```python
from build123d import *

# Parameters (mm, degrees)
SKETCH1_R           = 3.5
SKETCH1_R_2         = 1.5
BOSS_EXTRUDE1_DEPTH = 2
FILLET2_R           = 5
SKETCH2_R           = 5.5
SKETCH2_R_2         = 1.235500329
BOSS_EXTRUDE2_DEPTH = 5
FILLET3_R           = 2
CUT_EXTRUDE1_START  = -5
SKETCH3_R           = 3
CUT_EXTRUDE1_DEPTH  = 4


with BuildPart() as part:
    # Sketch1 → Boss-Extrude1 (new body)
    with BuildSketch(Plane(origin=(0, 0, 0), x_dir=(1, 0, 0), z_dir=(0, 1, 0))):
        Polygon((0, 6.5), (-22.384997637, 4.939274727), (-22.384997637, -5.060725273), (0, -6.5), (21.514033914, -5), (21.514033914, 5), align=None)
        with Locations(Location((0, 0, 0), (0, 0, 270))):
            Circle(SKETCH1_R, mode=Mode.SUBTRACT)
        with Locations(Location((-18, 0, 0), (0, 0, 270))):
            Circle(SKETCH1_R_2, mode=Mode.SUBTRACT)
        with Locations(Location((18, 0, 0), (0, 0, 270))):
            Circle(SKETCH1_R_2, mode=Mode.SUBTRACT)
    extrude(amount=BOSS_EXTRUDE1_DEPTH)

    # Fillet2
    fillet2_edges = [part.edges().sort_by_distance(p)[0] for p in [
        (-22.384997637, 1, 5.060725273),
        (-22.384997637, 1, -4.939274727),
        (21.514033914, 1, -5),
        (21.514033914, 1, 5),
    ]]
    fillet(fillet2_edges, radius=FILLET2_R)

    # Sketch2 → Boss-Extrude2 (add)
    with BuildSketch(Plane(origin=(0, 0, 0), x_dir=(1, 0, 0), z_dir=(0, 1, 0))):
        with Locations(Location((0, 0, 0), (0, 0, 270))):
            Circle(SKETCH2_R)
        with Locations(Location((0, 0, 0), (0, 0, 270))):
            Circle(SKETCH2_R_2, mode=Mode.SUBTRACT)
    extrude(amount=-BOSS_EXTRUDE2_DEPTH)

    # Fillet3
    # the kernel refuses this fillet: 2 mm, written as the material it adds along each edge
    with BuildSketch(Plane(origin=(0, 0, 0), x_dir=(0, 0, 1), z_dir=(-1, 0, 0))) as fillet3_piece_1_section:
        with BuildLine():
            CenterArc((5.5 + FILLET3_R, -FILLET3_R), FILLET3_R, 90, 90)
            Line((5.5, -FILLET3_R), (5.5, 0))
            Line((5.5, 0), (5.5 + FILLET3_R, 0))
        make_face()
    fillet3_piece_1 = revolve(axis=Axis((0, 0, 0), (0, 1, 0)), mode=Mode.PRIVATE)
    fillet3_piece_1 = split(fillet3_piece_1, bisect_by=Plane(origin=(-0.030373147, -0.562249721, -6.497882326), z_dir=(0.06955308260096395, 0, 0.9975782519184666)), keep=Keep.TOP, mode=Mode.PRIVATE)
    fillet3_piece_1 = split(fillet3_piece_1, bisect_by=Plane(origin=(0.030373147, -0.562249721, -6.497882326), z_dir=(-0.06955308260096384, 0, 0.9975782519184666)), keep=Keep.TOP, mode=Mode.PRIVATE)
    fillet3_piece_1 = split(fillet3_piece_1, bisect_by=Plane(origin=(-0.804382076, -0.562249721, 6.44828113), z_dir=(0.06416390756024656, 0, -0.9979393733922919)), keep=Keep.TOP, mode=Mode.PRIVATE)
    fillet3_piece_1 = split(fillet3_piece_1, bisect_by=Plane(origin=(0.871627207, -0.562249721, 6.439228468), z_dir=(-0.06955308260096384, 0, -0.9975782519184666)), keep=Keep.TOP, mode=Mode.PRIVATE)
    add(fillet3_piece_1)

    # Sketch3 → Cut-Extrude1 (cut)
    with BuildSketch(Plane(origin=(0, 0, 0), x_dir=(1, 0, 0), z_dir=(0, 1, 0)).offset(CUT_EXTRUDE1_START)):
        with Locations(Location((0, 0, 0), (0, 0, 270))):
            Circle(SKETCH3_R)
    extrude(amount=CUT_EXTRUDE1_DEPTH, mode=Mode.SUBTRACT)


solid = part.part
```
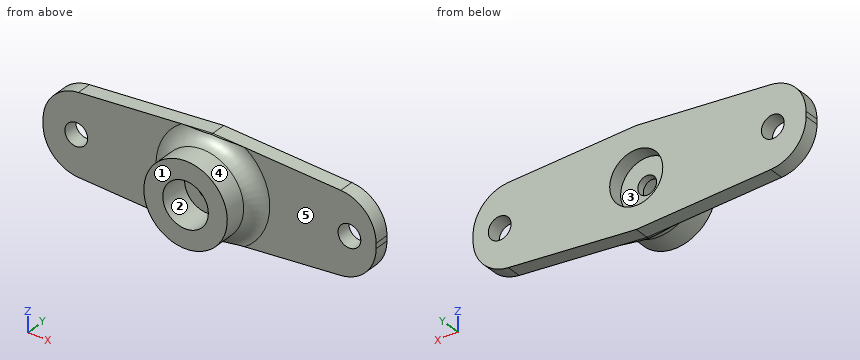
Could you check a few things on this model? Use its own coordinates, in mm. Face numbers are marked on the shaded views. A direction names the side the tool comes from. Give positions to 0.01 mm unless a question says otherwise; leave off trailing zeros. Write each loop counter-clockwise with the first axis right and the second up, starting at its lowest first coordinate (ties: lowest second). Pieces come first, ordered by that corner, then holes. Notation, with made-up numbers: (38.25, 17.5) -> (94.25, 17.5) arc R14 cw to (94.25, 42.5) -> close; hole circle Ø4 at (24.25, 31). An arc over 180 degrees is marked (long way). Write each question's results on one line, items separated by ' | '.
1. If we mould it in two halves opening along X, with no side actions, what happens to the marked faces 3, 4 and 5? For each: released by +X, released by -X, zero draft, split by the parting line, or undercut.
Check sheet entries:
face 3: undercut | face 4: split by the parting line | face 5: zero draft
2. Will these pins go through, and if not, where does the flat tip stop? pin 1 Ø6.5 at (x, z) = (0, 0) entering from -Y; pin 2 Ø2 at (x, y) = (16.5, -1.5) entering from -Z; pin 3 Ø5.5 at (x, z) = (0, 0) entering from -Y; pin 4 Ø4 at (x, z) = (0, 0) entering from +Y.
Check sheet entries:
pin 1: stops at y = -5 | pin 2: passes through | pin 3: stops at y = -1 | pin 4: stops at y = 0
3. I want a section at B-B, the plane x = -19. Write out the boundary of the cut face in (y, z).
Check sheet entries:
outline: (0, -5.01) -> (2, -5.01) -> (2, -1.12) -> (0, -1.12) -> close; (0, 1.12) -> (2, 1.12) -> (2, 5.1) -> (0, 5.1) -> close
4. I need wall thicknesses on L1, parallel to X at y = 0.5, z = 0 (3 decimals); L2, parallel to Y at x = -9, z = -1; L3, parallel to Z at x = -2, y = 1.25. Which ranges of each line are inside material? Lowest first, please.
Check sheet entries:
L1: x = -22.385 to -19.5, -16.5 to -3.5, 3.5 to 16.5, 19.5 to 21.514 | L2: y = 0 to 2 | L3: z = -6.36 to -2.87, 2.87 to 6.37
5. I want a section at C-C, the plane x = 18. Write out the boundary of the cut face in (y, z).
Check sheet entries:
outline: (0, -5.11) -> (2, -5.11) -> (2, -1.5) -> (0, -1.5) -> close; (0, 1.5) -> (2, 1.5) -> (2, 5.11) -> (0, 5.11) -> close
6. On a 3-axis mill with a long thin cutter (end or side, diameter ignored), from which of +Z, -Z, +X, -X, +Y, -Y can I reach the whole of each face in a straight line? I mean the marked faces 1 and 2. Say none if no direction works.
Check sheet entries:
face 1: +Z, -Z, +X, -X, -Y | face 2: -Y
7. I want a section at D-D, the plane x = 12.5. Write out the boundary of the cut face in (y, z).
Check sheet entries:
outline: (0, -5.63) -> (2, -5.63) -> (2, 5.63) -> (0, 5.63) -> close
8. I want a section at A-A, the plane y = 1. Write out the boundary of the cut face in (x, z) (3 decimals).
Check sheet entries:
outline: (-22.385, -0.276) arc R5 ccw to (-17.733, -5.264) -> (0, -6.5) -> (16.862, -5.324) arc R5 ccw to (21.514, -0.336) -> (21.514, 0.336) arc R5 ccw to (16.862, 5.324) -> (0, 6.5) -> (-17.706, 5.362) arc R5 ccw to (-22.385, 0.372) -> close; hole circle Ø3 at (-18, 0); hole circle Ø7 at (0, 0); hole circle Ø3 at (18, 0)
